Here's the drawing with two shaded views (mm, measured from the low corner). I have some questions. Give positions to 0.01 mm unless a question says otherwise; leave off trailing zeros. Order: outer loops, then holes, each group sorted by start corner. A loop starts at its lowest first (then second) coordinate and runs counter-clockwise, first axis right, second up. Notation, with made-up numbers: (48, 20) - (70, 20) arc R19 cw to (70, 26) - close; hole circle Ø1 at (-16, -18). An arc over 180 degrees is marked (long way). Use one line per item in the form item = value. Start each with the question number.
1) For pin 1 (3 mm diameter, centred on x = 19, z = 3.5, fed in from +Y) (1 decimal); pin 2 (1.9 mm diameter, centred on y = 67.5, z = 2, fed in from +X); pin 3 (3 mm diameter, centred on y = 111.5, z = 4, fed in from -X), each with a flat end and sliding along its axis, tell me the tip position at first contact or that it passes through.
2) Suppose I cut it at D-D, the plane x = 41. Write out the boundary of the cut face in (y, z).
3) Suppose I cut it at C-C, the plane y = 109. Write out the boundary of the cut face in (x, z).
4) Please list where these lines run through material, in increasing order: probe 1 along X at (y, z) = (64, 1) (1 decimal); probe 2 along Y at (x, z) = (20, 3.75); probe 3 along Y at (x, z) = (50, 3.25).
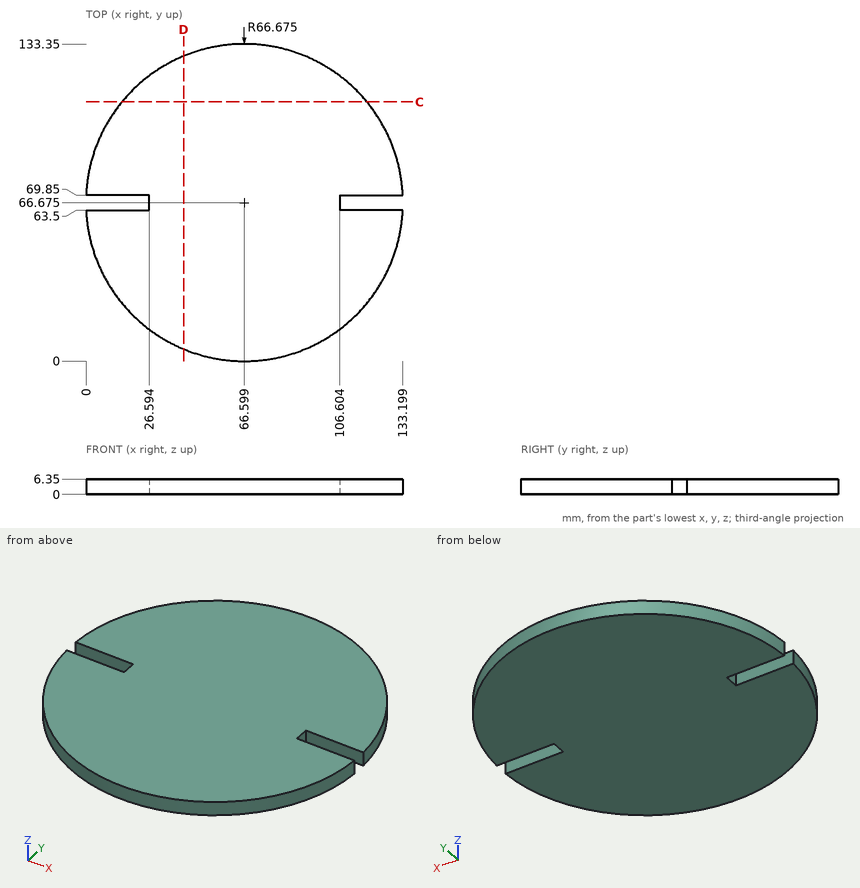
Result sheet:
q1.pin_1 = 114.8
q1.pin_2 = 106.6
q1.pin_3 = 15.92
q2.outline = (5.11, 0) - (128.24, 0) - (128.24, 6.35) - (5.11, 6.35) - close
q3.outline = (15.08, 0) - (118.12, 0) - (118.12, 6.35) - (15.08, 6.35) - close
q4.probe_1 = 26.6 to 106.6
q4.probe_2 = 18.99 to 63.5, 69.85 to 114.36
q4.probe_3 = 2.1 to 131.25
